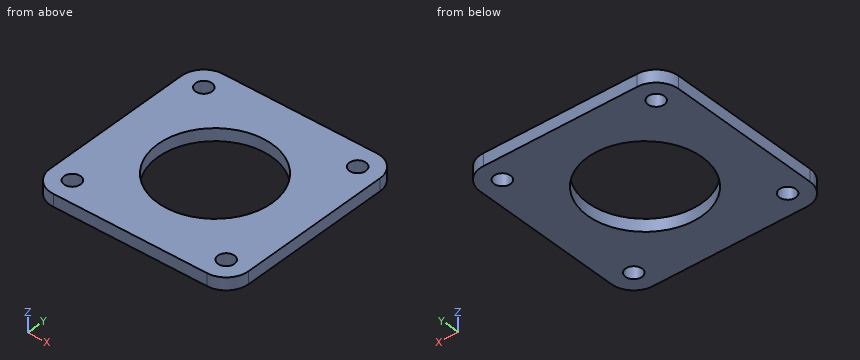
```python
from build123d import *

# Parameters (mm, degrees)
SKETCH_W   = 40
SKETCH_H   = 40
SKETCH_R   = 1.65
SKETCH_R_2 = 11.5
PAD_DEPTH  = 2.5
FILLET_R   = 4.5


with BuildPart() as part:
    # Sketch → Pad (new body)
    with BuildSketch(Plane.XY):
        Rectangle(SKETCH_W, SKETCH_H)
        with Locations((-15.5, 15.5)):
            Circle(SKETCH_R, mode=Mode.SUBTRACT)
        with Locations((15.5, 15.5)):
            Circle(SKETCH_R, mode=Mode.SUBTRACT)
        with Locations((15.5, -15.5)):
            Circle(SKETCH_R, mode=Mode.SUBTRACT)
        with Locations((-15.5, -15.5)):
            Circle(SKETCH_R, mode=Mode.SUBTRACT)
        Circle(SKETCH_R_2, mode=Mode.SUBTRACT)
    extrude(amount=PAD_DEPTH)

    # Fillet
    fillet_edges = [part.edges().sort_by_distance(p)[0] for p in [
        (-20, -20, 1.25),
        (-20, 20, 1.25),
        (20, 20, 1.25),
        (20, -20, 1.25),
    ]]
    fillet(fillet_edges, radius=FILLET_R)


solid = part.part
```
Geometry: final body of the model. Coordinates: model frame, mm. Round coordinates to 2 decimals unless told otherwise and drop trailing zeros. Loops run counter-clockwise (first coordinate to the right, second up) from the corner with the lowest first, then second, coordinate; pieces in that order, holes last. Notation, with made-up numbers: (85.25, 33.25) -> (133.25, 33.25) arc R21 cw to (133.25, 54.25) -> close; hole circle Ø11 at (72, 14.5). An arc over 180 degrees is marked (long way). Write each question's results on one line, items separated by ' | '.
Item 1: Cut plane D-D on y = 15. Return the cut outline in (x, z), and give its area (3 significant figures).
Answers below:
outline: (-20, 0) -> (-17.07, 0) -> (-17.07, 2.5) -> (-20, 2.5) -> close; (-13.93, 0) -> (13.93, 0) -> (13.93, 2.5) -> (-13.93, 2.5) -> close; (17.07, 0) -> (20, 0) -> (20, 2.5) -> (17.07, 2.5) -> close | area: 84.3 mm²
Item 2: Cut plane C-C on z = 1.35. Return the cut outline in (x, y), and give its area (3 significant figures).
Answers below:
outline: (-20, -15.5) arc R4.5 ccw to (-15.5, -20) -> (15.5, -20) arc R4.5 ccw to (20, -15.5) -> (20, 15.5) arc R4.5 ccw to (15.5, 20) -> (-15.5, 20) arc R4.5 ccw to (-20, 15.5) -> close; hole circle Ø3.3 at (-15.5, -15.5); hole circle Ø3.3 at (-15.5, 15.5); hole circle Ø23 at (0, 0); hole circle Ø3.3 at (15.5, -15.5); hole circle Ø3.3 at (15.5, 15.5) | area: 1,130 mm²
Item 3: Line query: probe 1 along Y at (x, z) = (15.5, 1.15); probe 2 along X at (y, z) = (-0.5, 0.75); probe 3 along X at (y, z) = (-17, 2.15). Output: solid intervals per line, ascending. Write a range as [from, to].
Answers below:
probe 1: y = [-20, -17.15], [-13.85, 13.85], [17.15, 20] | probe 2: x = [-20, -11.49], [11.49, 20] | probe 3: x = [-19.74, -16.19], [-14.81, 14.81], [16.19, 19.74]
Item 4: Cut plane A-A on y = 0. Return the cut outline in (x, z).
Answers below:
outline: (-20, 0) -> (-11.5, 0) -> (-11.5, 2.5) -> (-20, 2.5) -> close; (11.5, 0) -> (20, 0) -> (20, 2.5) -> (11.5, 2.5) -> close
Item 5: Pin query (flat end, axial travel): pin 1 Ø2.5 at (x, y) = (-15.5, 15.5) entering from +Z. Return the tip coordinate at first contact, or that it passes through.
Answers below:
pin 1: passes through
